from build123d import *

# Parameters (mm, degrees)
ESQUISSE1_R                  = 2
BOSS_EXTRU_1_DEPTH           = 3
BOSS_EXTRU_2_DEPTH           = 30
CONG_1_START                 = -11
CONG_1_DEPTH                 = 34
CONG_1_2_DEPTH               = 25
CONG_1_START_2               = 16.9999999
CONG_1_3_DEPTH               = 6.0000001
CONG_1_START_3               = 3
CONG_1_4_DEPTH               = 2
ENL_V_MAT_EXTRU_1_DEPTH      = 74.008561265
ENL_V_MAT_EXTRU_1_DEPTH_BACK = 74.008561265
ESQUISSE3_W                  = 37.381504973
ESQUISSE3_H                  = 48.316758503


with BuildPart() as part:
    # Esquisse1 → Boss.-Extru.1 (new body)
    with BuildSketch(Plane.XY):
        with BuildLine():
            Line((-5, 1.5), (23, 1.5))
            Line((23, 1.5), (23, 31.5))
            Line((23, 31.5), (-8, 31.5))
            ThreePointArc((-8, 31.5), (-10.121320344, 30.621320344), (-11, 28.5))
            Line((-11, 28.5), (-11, 7.5))
            ThreePointArc((-11, 7.5), (-9.242640687, 3.257359313), (-5, 1.5))
        make_face()
        with Locations((-5, 7.5)):
            Circle(ESQUISSE1_R, mode=Mode.SUBTRACT)
        with Locations((7.5, 7.5)):
            Circle(ESQUISSE1_R, mode=Mode.SUBTRACT)
        with BuildLine():
            Line((14, 23.5), (17, 23.5))
            ThreePointArc((17, 23.5), (19, 21.5), (17, 19.5))
            Line((17, 19.5), (14, 19.5))
            ThreePointArc((14, 19.5), (12, 21.5), (14, 23.5))
        make_face(mode=Mode.SUBTRACT)
    boss_extru_1 = extrude(amount=BOSS_EXTRU_1_DEPTH)

    # Esquisse2 → Boss.-Extru.2 (add)
    with BuildSketch(Plane.XY.offset(3)):
        with BuildLine():
            Line((23, 31.5), (-8, 31.5))
            ThreePointArc((-8, 31.5), (-10.121320344, 30.621320344), (-11, 28.5))
            Line((-11, 28.5), (-11, 26.5))
            Line((-11, 26.5), (23, 26.5))
            Line((23, 26.5), (23, 31.5))
        make_face()
    boss_extru_2 = extrude(amount=BOSS_EXTRU_2_DEPTH)

    # Congé1: read off the stored shape, not the designer's step
    # Congé1 outline → Congé1 (add)
    with BuildSketch(Plane.YZ.offset(CONG_1_START)):
        with BuildLine():
            ThreePointArc((26.5, 9), (25.696152423, 6), (23.5, 3.803847577))
            Line((23.5, 3.803847577), (23.5, 3))
            Line((23.5, 3), (26.5, 3))
            Line((26.5, 3), (26.5, 9))
        make_face()
    cong_1 = extrude(amount=CONG_1_DEPTH)

    # Cong_1 2 outline → Cong_1 2 (add)
    with BuildSketch(Plane.YZ.offset(CONG_1_START)):
        with BuildLine():
            Line((23.5, 3), (23.5, 3.803847577))
            ThreePointArc((23.5, 3.803847577), (22.052914271, 3.204445042), (20.5, 3))
            Line((20.5, 3), (23.5, 3))
        make_face()
    cong_1_2 = extrude(amount=CONG_1_2_DEPTH)

    # Cong_1 3 outline → Cong_1 3 (add)
    with BuildSketch(Plane.YZ.offset(CONG_1_START_2)):
        with BuildLine():
            Line((23.5, 3), (23.5, 3.803847577))
            ThreePointArc((23.5, 3.803847577), (22.052914271, 3.204445042), (20.5, 3))
            Line((20.5, 3), (23.5, 3))
        make_face()
    cong_1_3 = extrude(amount=CONG_1_3_DEPTH)

    # Cong_1 4 outline → Cong_1 4 (cut)
    with BuildSketch(Plane.XY.offset(CONG_1_START_3)):
        with BuildLine():
            Line((17, 23.5), (17, 19.5))
            ThreePointArc((17, 19.5), (19, 21.5), (17, 23.5))
        make_face()
        with BuildLine():
            ThreePointArc((14, 23.5), (12, 21.5), (14, 19.5))
            Line((14, 19.5), (14, 23.5))
        make_face()
    cong_1_4 = extrude(amount=CONG_1_4_DEPTH, mode=Mode.SUBTRACT)

    # Symétrie1: Boss.-Extru.1, Boss.-Extru.2, Congé1, Cong_1 2, Cong_1 3, Cong_1 4 across plane
    add(boss_extru_1.mirror(Plane(origin=(23, 1.5, 3), x_dir=(0, 0, 1), z_dir=(-1, 0, 0))))
    add(boss_extru_2.mirror(Plane(origin=(23, 1.5, 3), x_dir=(0, 0, 1), z_dir=(-1, 0, 0))))
    add(cong_1.mirror(Plane(origin=(23, 1.5, 3), x_dir=(0, 0, 1), z_dir=(-1, 0, 0))))
    add(cong_1_2.mirror(Plane(origin=(23, 1.5, 3), x_dir=(0, 0, 1), z_dir=(-1, 0, 0))))
    add(cong_1_3.mirror(Plane(origin=(23, 1.5, 3), x_dir=(0, 0, 1), z_dir=(-1, 0, 0))))
    add(cong_1_4.mirror(Plane(origin=(23, 1.5, 3), x_dir=(0, 0, 1), z_dir=(-1, 0, 0))), mode=Mode.SUBTRACT)

    # Esquisse3 → Enlèv. mat.-Extru.1 (cut, two sides: drawn at the far end of the back side and taken through both)
    with BuildSketch(Plane.XY.offset(33).offset(-ENL_V_MAT_EXTRU_1_DEPTH_BACK)):
        with Locations((4.309247513, 15.68567261)):
            Rectangle(ESQUISSE3_W, ESQUISSE3_H)
    extrude(amount=ENL_V_MAT_EXTRU_1_DEPTH + ENL_V_MAT_EXTRU_1_DEPTH_BACK, mode=Mode.SUBTRACT)


solid = part.part
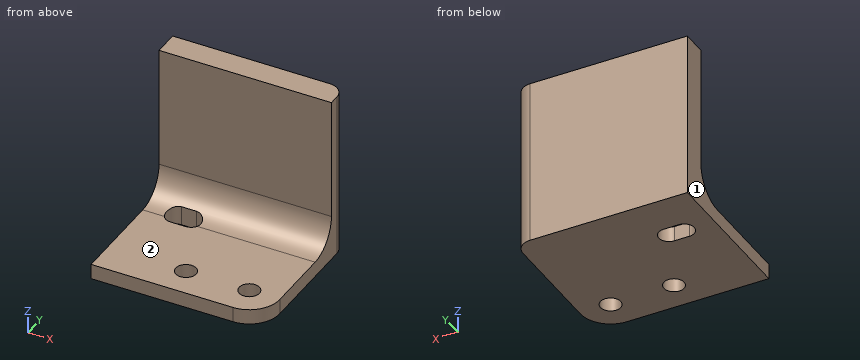
The listing builds one solid part. Answer for the finished solid, in the listing's coordinates (mm). Face numbers are marked on the shaded views. A direction names the side the tool comes from. Coordinates: 2 decimals unless noted, no trailing zeros. Loops run counter-clockwise (first coordinate to the right, second up) from the corner with the lowest first, then second, coordinate; pieces in that order, holes last.
1) Find section A-A on x = 39. Write down the section's boundary in (y, z).
2) A tool of negligible diameter and unlimited length cuts with its end or side. For the marked faces 1 and 2, from which of +Z, -Z, +X, -X, +Y, -Y can it reach the whole face along a straight path? Write none if from no direction.
3) Find section D-D on z = 30.5. Write down the section's boundary in (x, y).
4) Find section B-B on y = 21.5. Write down the section's boundary in (x, z).
5) Flat-ended cylindrical pins translate along their axes: pin 1 Ø9.5 at (x, y) = (42, 10.5) entering from +Z; pin 2 Ø12 at (x, z) = (39.5, 20) entering from -Y. Find the tip coordinate at first contact, or state that the pin passes through.
6) Find the intervals of material crossed by L1, parallel to Y at x = 51, z = 1.1; L2, parallel to X at y = 7, z = 2; L3, parallel to Y at x = 50.5, z = 29.5, in increasing order.
7) Find section C-C on x = 45.5. Write down the section's boundary in (y, z), then the cut area to 3 significant figures.
Values:
1. outline: (1.5, 0) - (5.56, 0) - (5.56, 3) - (1.5, 3) - close; (9.44, 0) - (31.5, 0) - (31.5, 33) - (26.5, 33) - (26.5, 9) arc R6 cw to (20.5, 3) - (9.44, 3) - close
2. face 1: +Z, -Z, -X, +Y, -Y
2. face 2: +Z, +X, -X, -Y
3. outline: (23, 26.5) - (57, 26.5) - (57, 28.5) arc R3 ccw to (54, 31.5) - (23, 31.5) - close
4. outline: (23, 0) - (27, 0) - (27, 3.08) - (23, 3.08) - close; (34, 0) - (57, 0) - (57, 3.08) - (34, 3.08) - close
5. pin 1: stops at z = 3
5. pin 2: stops at y = 26.5
6. L1: y = 1.5 to 5.5, 9.5 to 31.5
6. L2: x = 23 to 36.56, 40.44 to 49.06, 52.94 to 56.98
6. L3: y = 26.5 to 31.5
7. outline: (1.5, 0) - (31.5, 0) - (31.5, 33) - (26.5, 33) - (26.5, 9) arc R6 cw to (20.5, 3) - (1.5, 3) - close
7. area: 248 mm2
